Read the model definition and answer for the solid it produces. Units are mm, in the model's axes. A direction names the side the tool comes from. Coordinates: 2 decimals unless noted, no trailing zeros. Write each loop counter-clockwise with the first axis right and the second up, starting at its lowest first coordinate (ties: lowest second). Pieces come first, ordered by that corner, then holes. Notation, with made-up numbers: (23, 54) - (52, 54) arc R35 cw to (52, 86) - close; hole circle Ø5 at (13.5, 83). An arc over 180 degrees is marked (long way). Use a Markdown table: item, result.
from build123d import *

# Parameters (mm, degrees)
BOSS_EXTRUDE1_DEPTH                             = 8
CUT_EXTRUDE1_REACH                              = 65.856
SKETCH4_W                                       = 55.8
SKETCH4_H                                       = 37.4
BOSS_EXTRUDE2_DEPTH                             = 37.4
BOSS_EXTRUDE3_DEPTH                             = 3
CUT_EXTRUDE2_START                              = -3
CUT_EXTRUDE2_DEPTH                              = 3
CUT_EXTRUDE3_START                              = -3
CUT_EXTRUDE3_DEPTH                              = 3
M4X0_7_TAPPED_HOLE1_D                           = 3.3
M4X0_7_TAPPED_HOLE1_DEPTH                       = 6
M4X0_7_TAPPED_HOLE1_TIP                         = 0.991420021
CSK_FOR_M4_FLAT_HEAD_MACHINE_SCREW1_D           = 4.8
CSK_FOR_M4_FLAT_HEAD_MACHINE_SCREW1_CSINK_D     = 9.4
CSK_FOR_M4_FLAT_HEAD_MACHINE_SCREW1_CSINK_ANGLE = 90
CBORE_FOR_M4_SHCS1_D                            = 4.8
CBORE_FOR_M4_SHCS1_CBORE_D                      = 8
CBORE_FOR_M4_SHCS1_CBORE_DEPTH                  = 3
M3X0_5_TAPPED_HOLE1_D                           = 2.5
M3X0_5_TAPPED_HOLE1_DEPTH                       = 4
M3X0_5_TAPPED_HOLE1_TIP                         = 0.751075774
FILLET1_R                                       = 6.35


with BuildPart() as part:
    # Sketch1 → Boss-Extrude1 (new body)
    with BuildSketch(Plane.XY.offset(8)):
        with BuildLine():
            Line((-23.45868709, 18.7), (-23.45868709, -18.7))
            ThreePointArc((-23.45868709, -18.7), (0, -30), (23.45868709, -18.7))
            Line((23.45868709, -18.7), (35.34131291, -18.7))
            Line((35.34131291, -18.7), (35.34131291, 18.7))
            Line((35.34131291, 18.7), (23.45868709, 18.7))
            ThreePointArc((23.45868709, 18.7), (0, 30), (-23.45868709, 18.7))
        make_face()
    extrude(amount=-BOSS_EXTRUDE1_DEPTH)

    # Sketch3 → Cut-Extrude1 (cut, up to next)
    with BuildSketch(Plane(origin=(-20.45868709, 0, 0), x_dir=(0, 0, -1), z_dir=(1, 0, 0)), mode=Mode.PRIVATE) as cut_extrude1_sk1:
        with BuildLine():
            Line((-8, 18.7), (-8, -18.7))
            ThreePointArc((-8, -18.7), (-0.254206384, 0), (-8, 18.7))
        make_face()
    cut_extrude1_tool1 = extrude(cut_extrude1_sk1.sketch, amount=-CUT_EXTRUDE1_REACH, mode=Mode.PRIVATE) & part.part
    add(cut_extrude1_tool1.solids().sort_by_distance((-20.458687, 0, 4.859168))[0], mode=Mode.SUBTRACT)

    # Sketch4 → Boss-Extrude2 (add)
    with BuildSketch(Plane.XY.offset(8)):
        with Locations((7.44131291, 0)):
            Rectangle(SKETCH4_W, SKETCH4_H)
    extrude(amount=BOSS_EXTRUDE2_DEPTH)

    # Sketch5 → Boss-Extrude3 (add)
    with BuildSketch(Plane.ZY.offset(20.45868709)):
        with BuildLine():
            Line((45.4, 18.7), (45.4, -18.7))
            Line((45.4, -18.7), (21.171890016, -18.7))
            ThreePointArc((21.171890016, -18.7), (7.2, 0), (21.171890016, 18.7))
            Line((21.171890016, 18.7), (45.4, 18.7))
        make_face()
    extrude(amount=BOSS_EXTRUDE3_DEPTH)

    # Sketch6 → Cut-Extrude2 (cut)
    with BuildSketch(Plane.ZY.offset(23.45868709).offset(CUT_EXTRUDE2_START)):
        with BuildLine():
            Line((45.4, -18.7), (45.4, -5.528109984))
            ThreePointArc((45.4, -5.528109984), (40.488582233, -13.788582233), (32.228109984, -18.7))
            Line((32.228109984, -18.7), (45.4, -18.7))
        make_face()
    extrude(amount=CUT_EXTRUDE2_DEPTH, mode=Mode.SUBTRACT)

    # Sketch7 → Cut-Extrude3 (cut)
    with BuildSketch(Plane.ZY.offset(23.45868709).offset(CUT_EXTRUDE3_START)):
        with BuildLine():
            Line((45.4, 18.7), (32.228109984, 18.7))
            ThreePointArc((32.228109984, 18.7), (40.488582233, 13.788582233), (45.4, 5.528109984))
            Line((45.4, 5.528109984), (45.4, 18.7))
        make_face()
    extrude(amount=CUT_EXTRUDE3_DEPTH, mode=Mode.SUBTRACT)

    # Sketch8 → Cut-Revolve1 (revolve, cut)
    with BuildSketch(Plane.XY.offset(26.7)):
        Polygon((-23.45868709, 15.86865), (-23.45868709, 0), (35.34131291, 0), (35.34131291, 15.86865), (9.94131291, 15.86865), (9.94131291, 13.5), (1.94131291, 13.5), (1.94131291, 15.86865), align=None)
    revolve(axis=Axis((-23.45868709, 0, 26.7), (1, 0, 0)), mode=Mode.SUBTRACT)

    # M4x0.7 Tapped Hole1
    with Locations(Plane(origin=(0, -18.7, 0), x_dir=(-1, 0, 0), z_dir=(0, -1, 0))):
        with Locations((12.45868709, -39.4), (-29.44131291, -39.4), (-29.44131291, -5.9)):
            Hole(M4X0_7_TAPPED_HOLE1_D / 2, depth=M4X0_7_TAPPED_HOLE1_DEPTH)
            with Locations((0, 0, -(M4X0_7_TAPPED_HOLE1_DEPTH + M4X0_7_TAPPED_HOLE1_TIP / 2))):  # 118° drill point
                Cone(0, M4X0_7_TAPPED_HOLE1_D / 2, M4X0_7_TAPPED_HOLE1_TIP, mode=Mode.SUBTRACT)

    # CSK for M4 Flat Head Machine Screw1 (through all)
    with Locations(Plane.XY.offset(8)):
        with Locations((0, -25.5), (0, 25.5)):
            CounterSinkHole(CSK_FOR_M4_FLAT_HEAD_MACHINE_SCREW1_D / 2, CSK_FOR_M4_FLAT_HEAD_MACHINE_SCREW1_CSINK_D / 2, counter_sink_angle=CSK_FOR_M4_FLAT_HEAD_MACHINE_SCREW1_CSINK_ANGLE)

    # CBORE for M4 SHCS1 (through all)
    with Locations(Plane.XY.offset(8)):
        with Locations((-12, -22.95), (12, -22.95), (12, 22.95), (-12, 22.95)):
            CounterBoreHole(CBORE_FOR_M4_SHCS1_D / 2, CBORE_FOR_M4_SHCS1_CBORE_D / 2, CBORE_FOR_M4_SHCS1_CBORE_DEPTH)

    # M3x0.5 Tapped Hole1
    with Locations(Plane.XY.offset(45.4)):
        with Locations((1.04131291, 8.07366885), (11.191713328, -14.199002102)):
            Hole(M3X0_5_TAPPED_HOLE1_D / 2, depth=M3X0_5_TAPPED_HOLE1_DEPTH)
            with Locations((0, 0, -(M3X0_5_TAPPED_HOLE1_DEPTH + M3X0_5_TAPPED_HOLE1_TIP / 2))):  # 118° drill point
                Cone(0, M3X0_5_TAPPED_HOLE1_D / 2, M3X0_5_TAPPED_HOLE1_TIP, mode=Mode.SUBTRACT)

    # Fillet1
    fillet1_edges = [part.edges().sort_by_distance(p)[0] for p in [
        (23.45868709, 18.7, 4),
        (23.45868709, -18.7, 4),
    ]]
    fillet(fillet1_edges, radius=FILLET1_R)


solid = part.part
(1) A cutting plane is placed at B-B, the plane z = 26.7. Write down the section's boundary in (x, y), and give its area (3 significant figures).
Report:
| item | result |
|---|---|
| outline | (-23.46, -18.7) - (35.34, -18.7) - (35.34, -15.87) - (9.94, -15.87) - (9.94, -13.5) - (1.94, -13.5) - (1.94, -15.87) - (-23.46, -15.87) - close; (-23.46, 15.87) - (1.94, 15.87) - (1.94, 13.5) - (9.94, 13.5) - (9.94, 15.87) - (35.34, 15.87) - (35.34, 18.7) - (-23.46, 18.7) - close |
| area | 371 mm² |
(2) Each of these flat-tipped pins is pushed along its axis until it touches: P1, Ø3, axis at x = -12.46, z = 39.4, coming from the +Y side; P2, Ø4.5, axis at x = -12, y = 22.95, coming from the -Z side; P3, Ø3, axis at x = -14, z = 19.5, coming from the -Y side; P4, Ø2.5, axis at x = 29.44, z = 39.4, coming from the -Y side. Where does it stop, or does it pass through?
Report:
| item | result |
|---|---|
| P1 | stops at y = 18.7 |
| P2 | passes through |
| P3 | stops at y = -18.7 |
| P4 | stops at y = -12.46 |
(3) The mould has two halves that part along Z. Classify faces 6 (the cylindrical face through (-10.9, -3.4, 11.2)), 7 (the cylindrical face through (-21.938, 13.884, 40.392)), 8 (the flat face through (6, 18.7, 27)): pulls with the +Z half, pulls with the -Z half, needs draft (parallel to the pull), parting line crosses it, or undercut.
Report:
| item | result |
|---|---|
| face 6 | undercut |
| face 7 | pulls with the +Z half |
| face 8 | needs draft |
(4) A cutting plane is placed at A-A, the plane y = 0. Write down the section's boundary in (x, z).
Report:
| item | result |
|---|---|
| outline | (-23.46, 0) - (35.34, 0) - (35.34, 10.83) - (9.94, 10.83) - (9.94, 13.2) - (1.94, 13.2) - (1.94, 10.83) - (-23.46, 10.83) - (-23.46, 7.2) - (-20.46, 7.2) - (-20.46, 0.25) - (-23.46, 0.25) - close; (-23.46, 42.57) - (1.94, 42.57) - (1.94, 40.2) - (9.94, 40.2) - (9.94, 42.57) - (35.34, 42.57) - (35.34, 45.4) - (-23.46, 45.4) - close |
(5) Straight lines are drawn through the part: L1, parallel to Y at x = -12, z = 5.75; L2, parallel to Y at x = -15, z = 7; L3, parallel to Z at x = -5.75, y = 0. For each, find the intervals that lie inside material, in ascending order.
Report:
| item | result |
|---|---|
| L1 | y = -27.5 to -26.95, -18.95 to 18.95, 26.95 to 27.5 |
| L2 | y = -25.98 to -25.6, -20.3 to 20.3, 25.6 to 25.98 |
| L3 | z = 0 to 10.83, 42.57 to 45.4 |
(6) For faces 1 (the flat face through (9.941, -11, 35)), 2 (the flat face through (-1, 20, 8)), 3 (the flat face through (-10, -25, 5)), 4 (the cylindrical face through (-21.938, -0.35, 7.203)), 5 (the cylindrical face through (-21.938, -13.692, 40.584)), determine the directions among +Z, -Z, +X, -X, +Y, -Y from which every point of the face is accessible in a straight line to the end or side of a thin tool.
Report:
| item | result |
|---|---|
| face 1 | +X |
| face 2 | +Z, +X, -X, +Y |
| face 3 | +Z |
| face 4 | -X |
| face 5 | +Z, -X, -Y |
(7) A cutting plane is placed at C-C, the plane x = 25. Write down the section's boundary in (y, z).
Report:
| item | result |
|---|---|
| outline | (-18.84, 0) - (18.84, 0) - (18.84, 8) - (18.7, 8) - (18.7, 45.4) - (-18.7, 45.4) - (-18.7, 8) - (-18.84, 8) - close; hole circle Ø31.74 at (0, 26.7) |
(8) A cutting plane is placed at D-D, the plane y = 12. Write down the section's boundary in (x, z), and give its area (3 significant figures).
Report:
| item | result |
|---|---|
| outline | (-23.46, 0) - (35.34, 0) - (35.34, 16.32) - (9.94, 16.32) - (9.94, 20.52) - (1.94, 20.52) - (1.94, 16.32) - (-23.46, 16.32) - (-23.46, 11.33) - (-20.46, 11.33) - (-20.46, 3.13) - (-23.46, 3.13) - close; (-23.46, 37.08) - (1.94, 37.08) - (1.94, 32.88) - (9.94, 32.88) - (9.94, 37.08) - (35.34, 37.08) - (35.34, 45.4) - (-20.46, 45.4) - (-20.46, 42.07) - (-23.46, 42.07) - close |
| area | 1,480 mm² |
